Input: dimensioned drawing with shaded views. Units: mm. Origin: part minimum x, y, z. A direction names the side the tool comes from. Coordinates: 2 decimals unless noted, no trailing zeros. Loops run counter-clockwise (first coordinate to the right, second up) from the corner with the lowest first, then second, coordinate; pieces in that order, holes last.
Item 1: Reachability of the marked faces 1, 2 and 3 from +Z, -Z, +X, -X, +Y, -Y: full face, straight path, thin tool, end or side. Return the list, or none.
Item 2: Pin query (flat end, axial travel): pin 1 Ø4 at (x, y) = (18, 7) entering from +Z; pin 2 Ø0.8 at (y, z) = (6.5, 5.5) entering from -X; pin 3 Ø3 at (x, y) = (12.5, 3.5) entering from -Z. Return the tip coordinate at first contact, or that it passes through.
Item 3: Line query: probe 1 along Y at (x, z) = (24, 0.8); probe 2 along Z at (x, y) = (24.5, 4.5); probe 3 along Z at (x, y) = (13.5, 7.75). Output: solid intervals per line, ascending.
Item 4: Section query C-C, the plane z = 4.5. Return the cut outline in (x, y), then the cut area to 3 significant figures.
Item 5: Pull-direction query (X, two-part tool) for the marked faces 4, 5 and 6; classes: +X half, -X half, draft (parallel to the pull), parting line (faces both ways), or undercut.
Item 6: Section query B-B, the plane y = 2. State how many separate pieces and enclosed holes the cut face has, then the cut area to 3 significant figures.
Item 7: Section query D-D, the plane x = 2. Return the cut outline in (y, z).
Item 8: Section query A-A, the plane x = 13. Return the cut outline in (y, z).
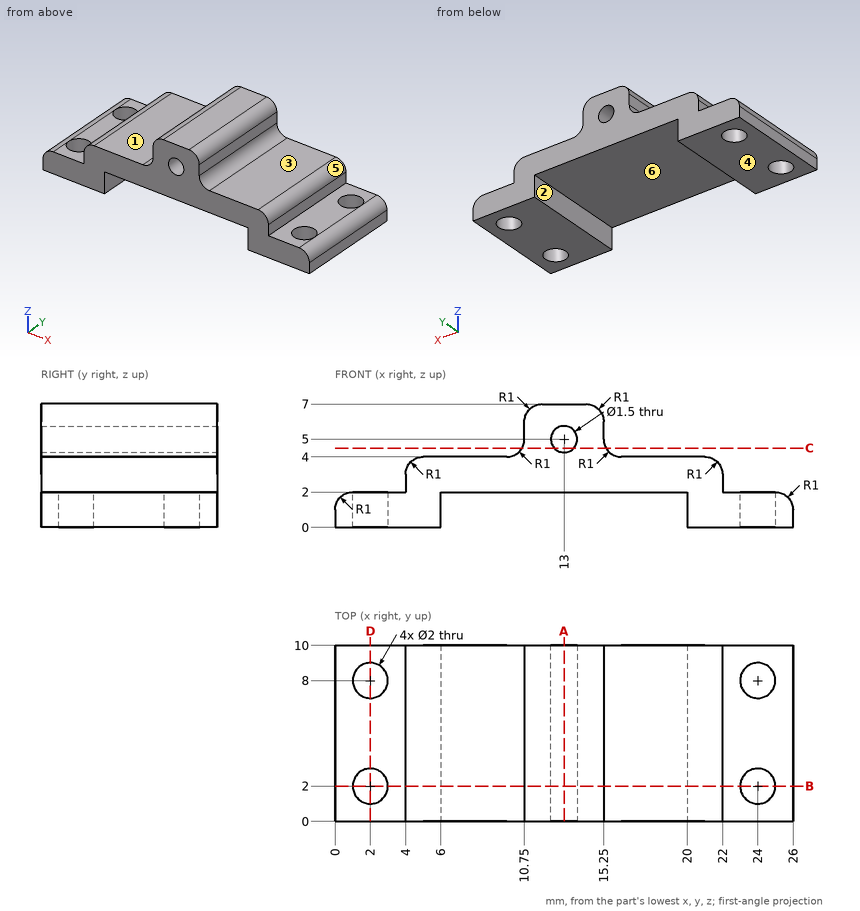
Verdict:
1. face 1: +Z, -X, +Y, -Y
1. face 2: -Z, +Y, -Y
1. face 3: +Z, +X, +Y, -Y
2. pin 1: stops at z = 4.03
2. pin 2: stops at x = 10.75
2. pin 3: stops at z = 2
3. probe 1: y = 0 to 1, 3 to 7, 9 to 10
3. probe 2: z = 0 to 2
3. probe 3: z = 2 to 4.44, 5.56 to 7
4. outline: (10.62, 0) - (12.44, 0) - (12.44, 10) - (10.62, 10) - close; (13.56, 0) - (15.38, 0) - (15.38, 10) - (13.56, 10) - close
4. area: 36.5 mm2
5. face 4: draft
5. face 5: +X half
5. face 6: undercut
6. separate pieces: 3
6. enclosed holes: 1
6. area: 62.9 mm2
7. outline: (0, 0) - (1, 0) - (1, 2) - (0, 2) - close; (3, 0) - (7, 0) - (7, 2) - (3, 2) - close; (9, 0) - (10, 0) - (10, 2) - (9, 2) - close
8. outline: (0, 2) - (10, 2) - (10, 4.25) - (0, 4.25) - close; (0, 5.75) - (10, 5.75) - (10, 7) - (0, 7) - close
